Model file for the job. Use its own axes, mm. A direction names the side the tool comes from. Round coordinates to 2 decimals unless told otherwise and drop trailing zeros. Loops run counter-clockwise (first coordinate to the right, second up) from the corner with the lowest first, then second, coordinate; pieces in that order, holes last. Notation, with made-up numbers: (-22.5, -28.75) -> (32.5, -28.75) arc R20 cw to (32.5, -22.75) -> close; hole circle Ø4 at (35.5, 86.25). An arc over 180 degrees is marked (long way). Use a Markdown table: item, result.
from build123d import *

# Parameters (mm, degrees)
SKETCH002_R   = 42
SKETCH002_R_2 = 40
PAD001_DEPTH  = 12
SKETCH003_W   = 8
SKETCH003_H   = 12
POCKET_DEPTH  = 42.001


with BuildPart() as part:
    # Sketch002 → Pad001 (new body)
    with BuildSketch(Plane.XY):
        Circle(SKETCH002_R)
        Circle(SKETCH002_R_2, mode=Mode.SUBTRACT)
    extrude(amount=PAD001_DEPTH)

    # Sketch003 → Pocket (cut, through all)
    with BuildSketch(Plane.XZ):
        with Locations((0, 8)):
            Rectangle(SKETCH003_W, SKETCH003_H)
    extrude(amount=-POCKET_DEPTH, mode=Mode.SUBTRACT)


solid = part.part
Q1. Band-saw the part on B-B, the plane y = 0. Give the cut face in (x, z), plus the area to 3 significant figures.
Results list:
| item | result |
|---|---|
| outline | (-42, 0) -> (-40, 0) -> (-40, 12) -> (-42, 12) -> close; (40, 0) -> (42, 0) -> (42, 12) -> (40, 12) -> close |
| area | 48.0 mm² |
Q2. Band-saw the part on C-C, the plane z = 8.75. Give the cut face in (x, y), plus the area to 3 significant figures.
Results list:
| item | result |
|---|---|
| outline | (-4, 39.8) -> (-4, 41.81) arc R42 ccw (long way) to (4, 41.81) -> (4, 39.8) arc R40 cw (long way) to start |
| area | 499 mm² |
Q3. Pull direction X, two halves, no side cores. Call faces 3 (the face through (-0.2, -40.3, 12)), 4 (the face through (40.06, 12.62, 5.92)), 5 (the face through (4, 41, 7)): released by +X, released by -X, zero draft, split by the parting line, or undercut.
Results list:
| item | result |
|---|---|
| face 3 | zero draft |
| face 4 | split by the parting line |
| face 5 | undercut |
Q4. Flat gauge pins, fed straight in: pin 1 (6 mm diameter, centred on y = 21, z = 3.5, fed in from +X); pin 2 (1.5 mm diameter, centred on x = 16.5, z = 10, fed in from +Y); pin 3 (8 mm diameter, centred on x = -23, y = -26, fed in from +Z); pin 4 (0.7 mm diameter, centred on x = 1.5, y = 41, fed in from +Z). Where does each tip first touch, or does it go through?
Results list:
| item | result |
|---|---|
| pin 1 | stops at x = 37.95 |
| pin 2 | stops at y = 38.94 |
| pin 3 | passes through |
| pin 4 | stops at z = 2 |
Q5. Band-saw the part on A-A, the plane x = 0. Give the cut face in (y, z), plus the area to 3 significant figures.
Results list:
| item | result |
|---|---|
| outline | (-42, 0) -> (-40, 0) -> (-40, 12) -> (-42, 12) -> close; (40, 0) -> (42, 0) -> (42, 2) -> (40, 2) -> close |
| area | 28.0 mm² |
Q6. Tool access for faces 1 (the face through (0, 41, 2)), 2 (the face through (-8.67, -39.05, 5.92)): list every direction of +Z, -Z, +X, -X, +Y, -Y with a clear straight run to the whole face (end or side of a thin tool).
Results list:
| item | result |
|---|---|
| face 1 | +Z, +Y |
| face 2 | +Z, -Z |
Q7. Drill centre lines: L1, parallel to X at y = 0, z = 6.75; L2, parallel to X at y = -7.5, z = 9.75; L3, parallel to Y at x = -23, z = 2.5. Where is each one in solid material? Low to high. Write a range as from..to.
Results list:
| item | result |
|---|---|
| L1 | x = -42..-40, 40..42 |
| L2 | x = -41.32..-39.29, 39.29..41.32 |
| L3 | y = -35.14..-32.73, 32.73..35.14 |
